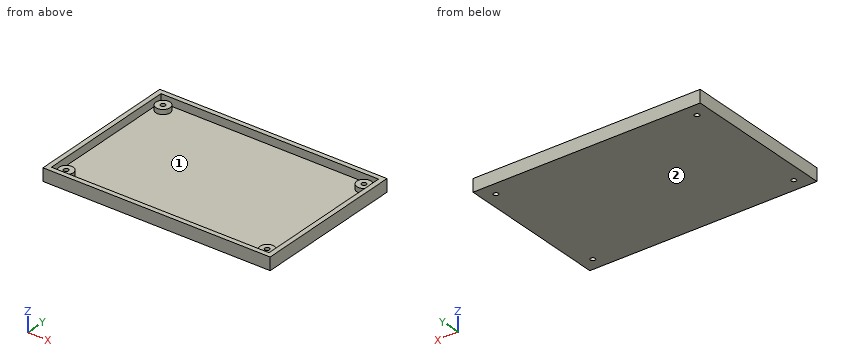
from build123d import *

# Parameters (mm, degrees)
SKETCH1_W           = 143.5
SKETCH1_H           = 96.5
SKETCH1_R           = 1.5
BOSS_EXTRUDE1_DEPTH = 8
SHELL1_T            = -3
SKETCH2_W           = 137.5
SKETCH2_H           = 90.5
CUT_EXTRUDE1_DEPTH  = 2


with BuildPart() as part:
    # Sketch1 → Boss-Extrude1 (new body)
    with BuildSketch(Plane.XY):
        with Locations((71.75, 48.25)):
            Rectangle(SKETCH1_W, SKETCH1_H)
        with Locations((8.5, 88)):
            Circle(SKETCH1_R, mode=Mode.SUBTRACT)
        with Locations((8.5, 8)):
            Circle(SKETCH1_R, mode=Mode.SUBTRACT)
        with Locations((135.5, 8)):
            Circle(SKETCH1_R, mode=Mode.SUBTRACT)
        with Locations((135.5, 88)):
            Circle(SKETCH1_R, mode=Mode.SUBTRACT)
    extrude(amount=BOSS_EXTRUDE1_DEPTH)

    # Shell1
    shell1_openings = [part.faces().sort_by_distance(p)[0] for p in [
        (71.75, 48.25, 8),
    ]]
    offset(amount=SHELL1_T, openings=shell1_openings, kind=Kind.INTERSECTION)

    # Sketch2 → Cut-Extrude1 (cut)
    with BuildSketch(Plane.XY.offset(8)):
        with Locations((71.75, 48.25)):
            Rectangle(SKETCH2_W, SKETCH2_H)
    extrude(amount=-CUT_EXTRUDE1_DEPTH, mode=Mode.SUBTRACT)


solid = part.part
The listing builds one solid part. Answer for the finished solid, in the listing's coordinates (mm). Face numbers are marked on the shaded views. Coordinates: 2 decimals unless noted, no trailing zeros. Write each loop counter-clockwise with the first axis right and the second up, starting at its lowest first coordinate (ties: lowest second). Pieces come first, ordered by that corner, then holes. Notation, with made-up numbers: (20, 9) - (43, 9) arc R11 ccw to (43, 30) - close; hole circle Ø10 at (-31, 60.5). An arc over 180 degrees is marked (long way). Return JSON: item names as keys, results as strings.
1. Consider line 1 along Y through (x, z) = (8.5, 2.85); line 2 along Y through (x, z) = (8.5, 3.1); line 3 along X through (y, z) = (8, 3.2). Determine where each line is inside the solid, lowest interval first.
Final values:
{"line 1": "0 to 6.5, 9.5 to 86.5, 89.5 to 96.5", "line 2": "0 to 3, 3.5 to 6.5, 9.5 to 12.5, 83.5 to 86.5, 89.5 to 92.5, 93.5 to 96.5", "line 3": "0 to 3, 4 to 7, 10 to 13, 131 to 134, 137 to 140, 140.5 to 143.5"}
2. The part is cut by section A-A on x = 135.5. Determine the outline of the cut face in (y, z), then the cut area to 4 significant figures.
Final values:
{"outline": "(0, 0) - (6.5, 0) - (6.5, 6) - (3.5, 6) - (3.5, 3) - (3, 3) - (3, 8) - (0, 8) - close; (9.5, 0) - (86.5, 0) - (86.5, 6) - (83.5, 6) - (83.5, 3) - (12.5, 3) - (12.5, 6) - (9.5, 6) - close; (89.5, 0) - (96.5, 0) - (96.5, 8) - (93.5, 8) - (93.5, 3) - (92.5, 3) - (92.5, 6) - (89.5, 6) - close", "area": "337.5 mm^2"}
3. The part is cut by section B-B on y = 8. Determine the outline of the cut face in (x, z).
Final values:
{"outline": "(0, 0) - (7, 0) - (7, 6) - (4, 6) - (4, 3) - (3, 3) - (3, 8) - (0, 8) - close; (10, 0) - (134, 0) - (134, 6) - (131, 6) - (131, 3) - (13, 3) - (13, 6) - (10, 6) - close; (137, 0) - (143.5, 0) - (143.5, 8) - (140.5, 8) - (140.5, 3) - (140, 3) - (140, 6) - (137, 6) - close"}
4. The part is cut by section C-C on y = 76.5. Determine the outline of the cut face in (x, z), then the cut area to 4 significant figures.
Final values:
{"outline": "(0, 0) - (143.5, 0) - (143.5, 8) - (140.5, 8) - (140.5, 3) - (3, 3) - (3, 8) - (0, 8) - close", "area": "460.5 mm^2"}
5. The part is cut by section D-D on x = 93. Determine the outline of the cut face in (y, z).
Final values:
{"outline": "(0, 0) - (96.5, 0) - (96.5, 8) - (93.5, 8) - (93.5, 3) - (3, 3) - (3, 8) - (0, 8) - close"}
6. Each of these flat-tipped pins is pushed along its axis until it touches: pin 1 Ø6 at (x, y) = (119, 21.5) entering from +Z; pin 2 Ø2.5 at (x, y) = (135.5, 88) entering from -Z; pin 3 Ø5 at (x, y) = (8.5, 88) entering from +Z. Where does it stop, or does it pass through?
Final values:
{"pin 1": "z = 3", "pin 2": "through", "pin 3": "z = 6"}
7. For a pull along X with two mould halves and no side action, classify the marked faces 1 and 2 as +X half, -X half, draft (parallel to the pull), parting line (faces both ways), or undercut.
Final values:
{"face 1": "undercut", "face 2": "draft"}
